Answer from the drawing. Dimensions are ordinates in mm from the lowest x, y and z of the part. A direction names the side the tool comes from. Give positions to 0.01 mm unless a question says otherwise; leave off trailing zeros. Write each loop counter-clockwise with the first axis right and the second up, starting at its lowest first coordinate (ties: lowest second). Pieces come first, ordered by that corner, then holes. Notation, with made-up numbers: (62, 80.5) -> (74, 80.5) arc R16 ccw to (74, 89.5) -> close; hole circle Ø8 at (38.5, 63.5). An arc over 180 degrees is marked (long way). Put each result on its own line as item: value. Start each with the question number.
1) A cutting plane is placed at D-D (x = 4.25). Write down the section's boundary in (y, z).
2) For the marked faces 5 and 6, determine the directions among +Z, -Z, +X, -X, +Y, -Y from which every point of the face is accessible in a straight line to the end or side of a thin tool.
3) A cutting plane is placed at C-C (y = 0.8). Write down the section's boundary in (x, z).
4) A cutting plane is placed at B-B (z = 17). Write down the section's boundary in (x, y).
5) Find the intervals of material crossed by line 1 along X through (y, z) = (1.4, 10); line 2 along X through (y, z) = (3.05, 10); line 3 along Y through (x, z) = (7.5, 15), in increasing order. Write a range as from..to.
6) A cutting plane is placed at A-A (x = 10). Write down the section's boundary in (y, z), then the cut area to 3 significant figures.
7) For a pull along Z with two mould halves and no side action, classify the marked faces 1, 2, 3 and 4 as released by +Z, released by -Z, zero draft, split by the parting line, or undercut.
8) Flat-ended cylindrical pins translate along their axes: pin 1 Ø3.5 at (x, z) = (10, 17) entering from +Y; pin 2 Ø1 at (y, z) = (2, 9) entering from -X; pin 3 Ø2.5 at (x, z) = (3, 10) entering from +Y; pin 4 Ø3 at (x, y) = (2.5, 2.5) entering from +Z. Find the tip coordinate at first contact, or state that the pin passes through.
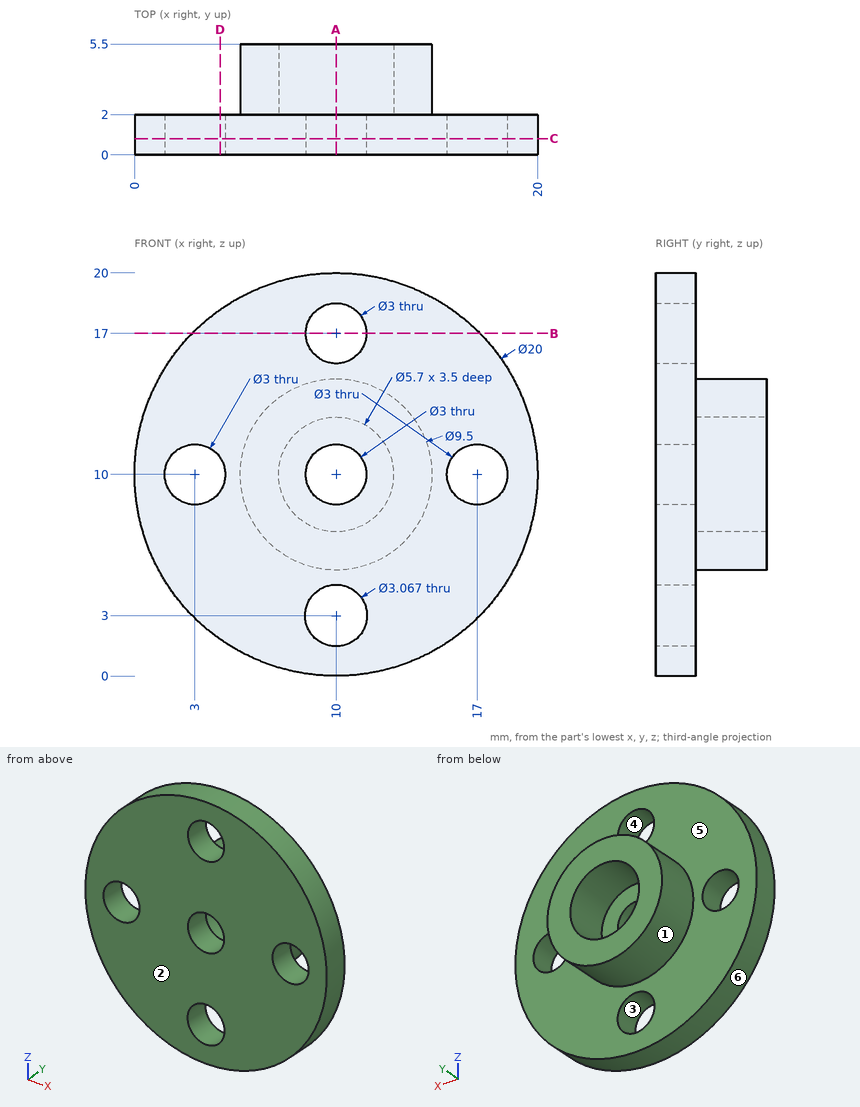
Reply:
1. outline: (0, 1.82) -> (2, 1.82) -> (2, 9.17) -> (0, 9.17) -> close; (0, 10.83) -> (2, 10.83) -> (2, 18.18) -> (0, 18.18) -> close
2. face 5: +Y
2. face 6: +Y, -Y
3. outline: circle Ø20 at (10, 10); hole circle Ø3 at (3, 10); hole circle Ø3.07 at (10, 3); hole circle Ø3 at (10, 10); hole circle Ø3 at (10, 17); hole circle Ø3 at (17, 10)
4. outline: (2.86, 0) -> (8.5, 0) -> (8.5, 2) -> (2.86, 2) -> close; (11.5, 0) -> (17.14, 0) -> (17.14, 2) -> (11.5, 2) -> close
5. line 1: x = 0..1.5, 4.5..8.5, 11.5..15.5, 18.5..20
5. line 2: x = 5.25..7.15, 12.85..14.75
5. line 3: y = 0..2
6. outline: (0, 0) -> (2, 0) -> (2, 1.47) -> (0, 1.47) -> close; (0, 4.53) -> (2, 4.53) -> (2, 5.25) -> (5.5, 5.25) -> (5.5, 7.15) -> (2, 7.15) -> (2, 8.5) -> (0, 8.5) -> close; (0, 11.5) -> (2, 11.5) -> (2, 12.85) -> (5.5, 12.85) -> (5.5, 14.75) -> (2, 14.75) -> (2, 15.5) -> (0, 15.5) -> close; (0, 18.5) -> (2, 18.5) -> (2, 20) -> (0, 20) -> close
6. area: 35.2 mm2
7. face 1: split by the parting line
7. face 2: zero draft
7. face 3: undercut
7. face 4: undercut
8. pin 1: stops at y = 2
8. pin 2: stops at x = 0.01
8. pin 3: passes through
8. pin 4: stops at z = 17.93
